The figure shows three views and two pictorial views of one solid part (mm, origin at its lowest corner). Answer the questions. Coordinates: 2 decimals unless noted, no trailing zeros. Write each loop counter-clockwise with the first axis right and the second up, starting at its lowest first coordinate (ties: lowest second). Pieces come first, ordered by that corner, then holes.
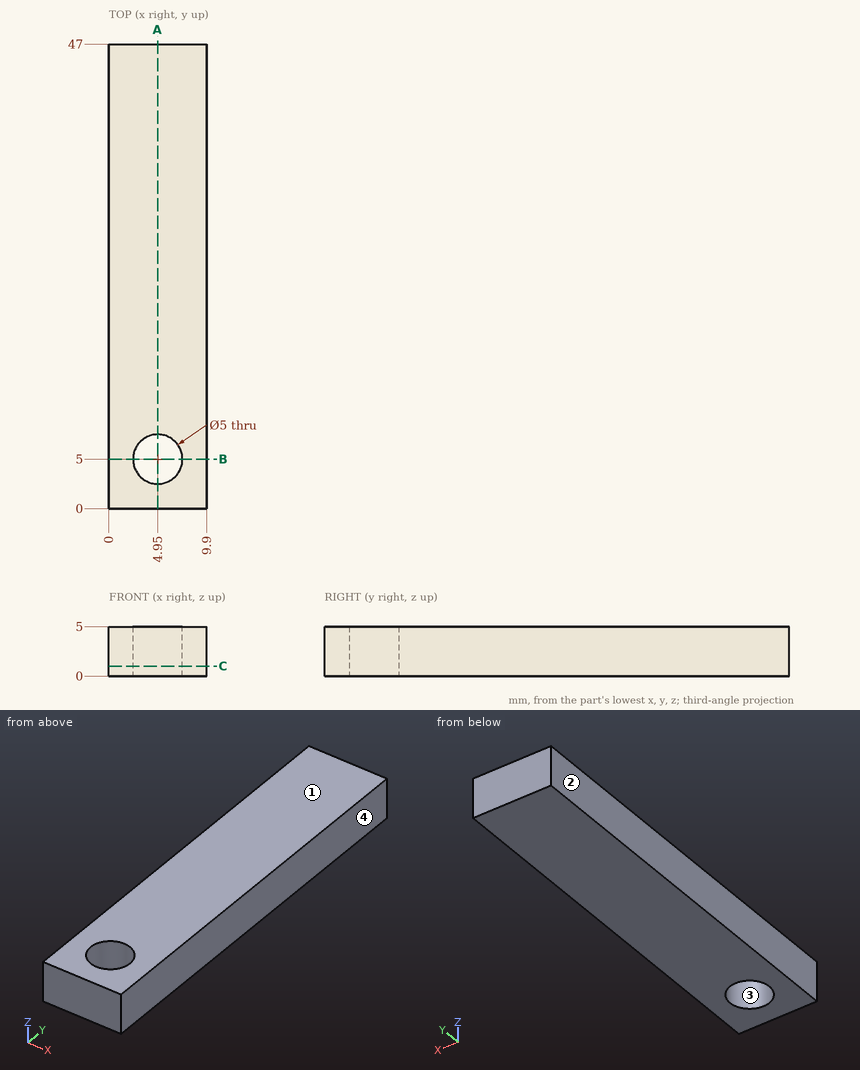
1. For a pull along X with two mould halves and no side action, classify the marked faces 1, 2, 3 and 4 as pulls with the +X half, pulls with the -X half, needs draft (parallel to the pull), parting line crosses it, or undercut.
Results found:
face 1: needs draft
face 2: pulls with the -X half
face 3: undercut
face 4: pulls with the +X half
2. Section A-A on x = 4.95 is taken. Give the vertices of the cut face in (y, z).
Results found:
outline: (0, 0) - (2.5, 0) - (2.5, 5) - (0, 5) - close; (7.5, 0) - (47, 0) - (47, 5) - (7.5, 5) - close
3. Find the intervals of material crossed by L1, parallel to Y at x = 4.95, z = 3.25; L2, parallel to Y at x = 6, z = 1.35, in increasing order.
Results found:
L1: y = 0 to 2.5, 7.5 to 47
L2: y = 0 to 2.73, 7.27 to 47
4. Flat-ended cylindrical pins translate along their axes: P1, Ø1, axis at x = 6.5, z = 1.5, coming from the -Y side; P2, Ø4, axis at x = 4.95, y = 5, coming from the +Z side. Find the tip coordinate at first contact, or state that the pin passes through.
Results found:
P1: stops at y = 0
P2: passes through
5. Section B-B on y = 5 is taken. Give the vertices of the cut face in (x, z), then the cut area to 3 significant figures.
Results found:
outline: (0, 0) - (2.45, 0) - (2.45, 5) - (0, 5) - close; (7.45, 0) - (9.9, 0) - (9.9, 5) - (7.45, 5) - close
area: 24.5 mm2
6. Section C-C on z = 1 is taken. Give the vertices of the cut face in (x, y).
Results found:
outline: (0, 0) - (9.9, 0) - (9.9, 47) - (0, 47) - close; hole circle Ø5 at (4.95, 5)
